The figure shows three views and two pictorial views of one solid part (mm, origin at its lowest corner). Answer the questions. Coordinates: 2 decimals unless noted, no trailing zeros. Write each loop counter-clockwise with the first axis right and the second up, starting at its lowest first coordinate (ties: lowest second). Pieces come first, ordered by that corner, then holes. Notation, with made-up numbers: (8.5, 13.5) -> (34.5, 13.5) arc R31 cw to (34.5, 50.5) -> close; hole circle Ø9 at (-31.75, 61). An arc over 180 degrees is marked (long way). Use CSV: the item, a comma, the result in double quotes. Start each with the question number.
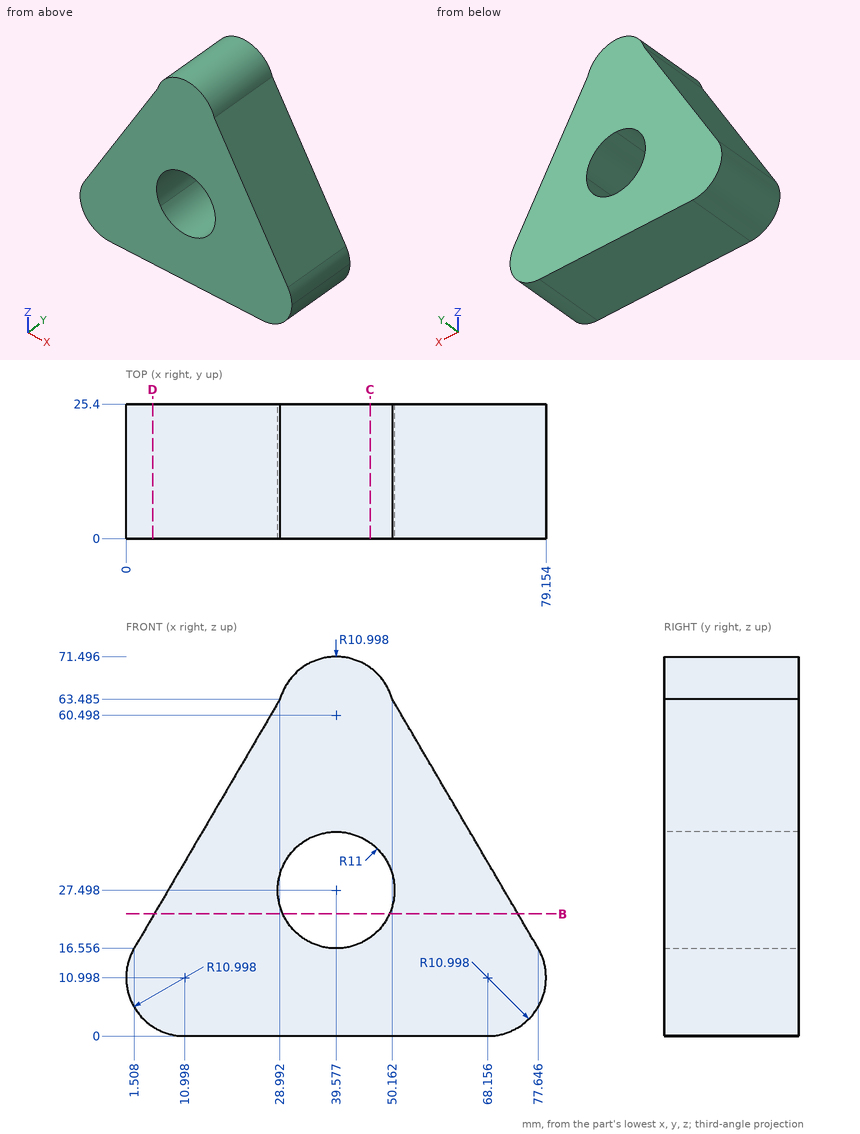
1) Section B-B, the plane z = 23 is taken. Give the vertices of the cut face in (x, y) (1 decimal).
2) Each of these flat-tipped pins is pushed along its axis until it touches: pin 1 (5 mm diameter, centred on y = 8.5, z = 55.5, fed in from -X); pin 2 (12 mm diameter, centred on x = 22, y = 15, fed in from +Z); pin 3 (3 mm diameter, centred on x = 16, y = 15.5, fed in from +Z). Where does it stop, or does it pass through?
3) Find the intervals of material crossed by line 1 along X through (y, z) = (10.5, 29) (1 decimal); line 2 along X through (y, z) = (11.25, 66) (1 decimal); line 3 along Z through (x, y) = (42, 13), in increasing order.
4) Section D-D, the plane x = 5 is taken. Give the vertices of the cut face in (y, z), plus the area to 3 significant figures.
5) Section C-C, the plane x = 46 is taken. Give the vertices of the cut face in (y, z).
The answers:
1,outline,"(5.3, 0) -> (29.5, 0) -> (29.5, 25.4) -> (5.3, 25.4) -> close; (49.6, 0) -> (73.9, 0) -> (73.9, 25.4) -> (49.6, 25.4) -> close"
2,pin 1,"stops at x = 22.85"
2,pin 2,"stops at z = 61.79"
2,pin 3,"stops at z = 43.86"
3,line 1,"x = 8.8 to 28.7, 50.5 to 70.4"
3,line 2,"x = 30.1 to 49.1"
3,line 3,"z = 0 to 16.77, 38.23 to 71.23"
4,outline,"(0, 1.78) -> (25.4, 1.78) -> (25.4, 22.52) -> (0, 22.52) -> close"
4,area,"527 mm^2"
5,outline,"(0, 0) -> (25.4, 0) -> (25.4, 18.57) -> (0, 18.57) -> close; (0, 36.43) -> (25.4, 36.43) -> (25.4, 69.43) -> (0, 69.43) -> close"
